```python
from build123d import *

# Parameters (mm, degrees)
CUT_EXTRUDE1_DEPTH = 3
CHAMFER1_SIZE      = 1


with BuildPart() as part:
    # Sketch1 → Revolve1 (revolve)
    with BuildSketch(Plane.XY):
        Polygon((-6, 0), (-6, 6.5), (0, 6.5), (0, 4), (15, 4), (15, 2.25), (17, 2.25), (17, 3), (24, 3), (24, 0), align=None)
    revolve(axis=Axis((-26.012554328, 0, 0), (1, 0, 0)))

    # Sketch2 → Cut-Extrude1 (cut)
    with BuildSketch(Plane.ZY.offset(6)):
        Polygon((2.886751346, 0), (1.443375673, 2.5), (-1.443375673, 2.5), (-2.886751346, 0), (-1.443375673, -2.5), (1.443375673, -2.5), align=None)
    extrude(amount=-CUT_EXTRUDE1_DEPTH, mode=Mode.SUBTRACT)

    # Chamfer1
    chamfer1_edges = [part.edges().sort_by_distance(p)[0] for p in [
        (-6, -6.5, 0),
    ]]
    chamfer(chamfer1_edges, length=CHAMFER1_SIZE)


solid = part.part
```
Could you check a few things on this model? Use its own coordinates, in mm. A direction names the side the tool comes from. Coordinates: 2 decimals unless noted, no trailing zeros. Order: outer loops, then holes, each group sorted by start corner. A loop starts at its lowest first (then second) coordinate and runs counter-clockwise, first axis right, second up. Notation, with made-up numbers: M -15,-13.75 L 12,-13.75 A17 ccw 12,-3.75 Z; hole C -11,43.5 d8. An arc over 180 degrees is marked long. Use one line per item in the form item = value. Start each with the question number.
1. Please list where these lines run through material, in increasing order: line 1 (X direction, y = -2.25, z = 1.75); line 2 (X direction, y = -0.5, z = 3); line 3 (X direction, y = 3, z = 3.5).
2. For pin 1 (6 mm diameter, centred on x = 15, z = 4.5, fed in from +Y); pin 2 (6 mm diameter, centred on x = 4.5, y = 2.5, fed in from +Z); pin 3 (1.5 mm diameter, centred on x = -2, z = -1, fed in from +Y), each with a flat end and sliding along its axis, tell me the tip position at first contact or that it passes through.
3. Suppose I cut it at B-B on x = 8.5. Write out the boundary of the cut face in (y, z).
4. On a 3-axis mill with a long thin cutter (end or side, diameter ignored), from which of +Z, -Z, +X, -X, +Y, -Y can I reach the whole of each face in a straight line? I mean faces 4 (the flat face through (-5, -2.5, 0)), 5 (the cylindrical face through (21, -3, 0)), 6 (the flat face through (15, 2, -2)). Say none if no direction works.
5. Suppose I cut it at A-A on z = 0. Write out the boundary of the cut face in (x, y).
6. We'd pull the mould along Z, two halves only. Please class faces 1 (the flat face through (-4.521, 1.233, 2.175)), 2 (the flat face through (-6, 3, 0)), 3 (the cylindrical face through (7.605, -0.867, -3.905)): +Z half, -Z half, draft (parallel to the pull), parting line (faces both ways), or undercut.
7. Suppose I cut it at C-C on x = 18.5. Write out the boundary of the cut face in (y, z), then the cut area to 3 significant figures.
Geometry says:
q1.line_1 = -6 to 15, 17 to 24
q1.line_2 = -6 to 15
q1.line_3 = -6 to 0
q2.pin_1 = 3.71
q2.pin_2 = 4
q2.pin_3 = 6.5
q3.outline = C 0,0 d8
q4.face_4 = -X
q4.face_5 = +X
q4.face_6 = none
q5.outline = M -6,-5.5 L -5,-6.5 L 0,-6.5 L 0,-4 L 15,-4 L 15,-2.25 L 17,-2.25 L 17,-3 L 24,-3 L 24,3 L 17,3 L 17,2.25 L 15,2.25 L 15,4 L 0,4 L 0,6.5 L -5,6.5 L -6,5.5 L -6,2.5 L -3,2.5 L -3,-2.5 L -6,-2.5 Z
q6.face_1 = undercut
q6.face_2 = draft
q6.face_3 = parting line
q7.outline = C 0,0 d6
q7.area = 28.3 mm^2
